Source: CAD feature listing. Evaluate the final solid. Frame: model axes, mm. Face numbers are marked on the shaded views. A direction names the side the tool comes from. Give positions to 0.01 mm unless a question says otherwise; leave off trailing zeros. Order: outer loops, then holes, each group sorted by start corner. A loop starts at its lowest first (then second) coordinate and runs counter-clockwise, first axis right, second up. Notation, with made-up numbers: (4, 61) - (35, 61) arc R26 ccw to (35, 81) - close; hole circle Ø4 at (56.25, -15.75). An arc over 180 degrees is marked (long way). Answer as CSV lines item,"result".
```python
from build123d import *
from build123d import SkipClean  # not in build123d's __all__

# Parameters (mm, degrees)
F3_DEPTH = 3.175
F4_DEPTH = 31.75
F5_DEPTH = 3.175
F6_DEPTH = 3.175


# Not quite as in the source:
# - a length typed as a fraction of an inch, garbled in the dataset ("3 / 203.2 mm" for 3/8 in), is restored


with BuildPart() as f3:
    # F2 (on Front) → F3 (new body)
    with BuildSketch(Plane.XZ):
        with BuildLine():
            Line((-3.175, 23.5998841364), (-3.175, 20.3918067186))
            ThreePointArc((-3.175, 20.3918067186), (-1.5922460699, 20.5759849996), (0, 20.6375))
            Line((0, 20.6375), (0, 23.8125))
            ThreePointArc((0, 23.8125), (-1.591055507, 23.7592865765), (-3.175, 23.5998841364))
        make_face()
        with BuildLine():
            ThreePointArc((20.6375, 0), (-13.4235305294, -15.6753065161), (-3.175, 20.3918067186))
            Line((-3.175, 20.3918067186), (-3.175, 23.5998841364))
            ThreePointArc((-3.175, 23.5998841364), (-15.6753065161, -17.9253987926), (23.8125, 0))
            ThreePointArc((23.8125, 0), (16.837980227, 16.837980227), (0, 23.8125))
            Line((0, 23.8125), (0, 20.6375))
            ThreePointArc((0, 20.6375), (14.5929161967, 14.5929161967), (20.6375, 0))
        make_face()
    extrude(amount=-F3_DEPTH)

    # F2 (on Front) → F4 (join)
    with BuildSketch(Plane.XZ):
        with BuildLine():
            ThreePointArc((0, 20.6375), (-1.5922460699, 20.5759849996), (-3.175, 20.3918067186))
            ThreePointArc((-3.175, 20.3918067186), (-13.4235305294, -15.6753065161), (20.6375, 0))
            ThreePointArc((20.6375, 0), (14.5929161967, 14.5929161967), (0, 20.6375))
        make_face()
    extrude(amount=F4_DEPTH)

    # F2 (on Front) → F5 (join)
    with BuildSketch(Plane.XZ):
        with BuildLine():
            Line((-3.175, 23.5998841364), (-3.175, 20.3918067186))
            ThreePointArc((-3.175, 20.3918067186), (-1.5922460699, 20.5759849996), (0, 20.6375))
            Line((0, 20.6375), (0, 23.8125))
            ThreePointArc((0, 23.8125), (-1.591055507, 23.7592865765), (-3.175, 23.5998841364))
        make_face()
    with SkipClean():  # cleaning this boolean's faces spoils the solid; the shape is the same uncleaned
        extrude(amount=F5_DEPTH)

    # F2 (on Front) → F6 (join)
    with BuildSketch(Plane.XZ):
        with BuildLine():
            ThreePointArc((0, 20.6375), (-1.5922460699, 20.5759849996), (-3.175, 20.3918067186))
            ThreePointArc((-3.175, 20.3918067186), (-13.4235305294, -15.6753065161), (20.6375, 0))
            ThreePointArc((20.6375, 0), (14.5929161967, 14.5929161967), (0, 20.6375))
        make_face()
        with BuildLine():
            Line((-3.175, 23.5998841364), (-3.175, 20.3918067186))
            ThreePointArc((-3.175, 20.3918067186), (-1.5922460699, 20.5759849996), (0, 20.6375))
            Line((0, 20.6375), (0, 23.8125))
            ThreePointArc((0, 23.8125), (-1.591055507, 23.7592865765), (-3.175, 23.5998841364))
        make_face()
    with SkipClean():  # cleaning this boolean's faces spoils the solid; the shape is the same uncleaned
        extrude(amount=-F6_DEPTH)


solid = f3.part
```
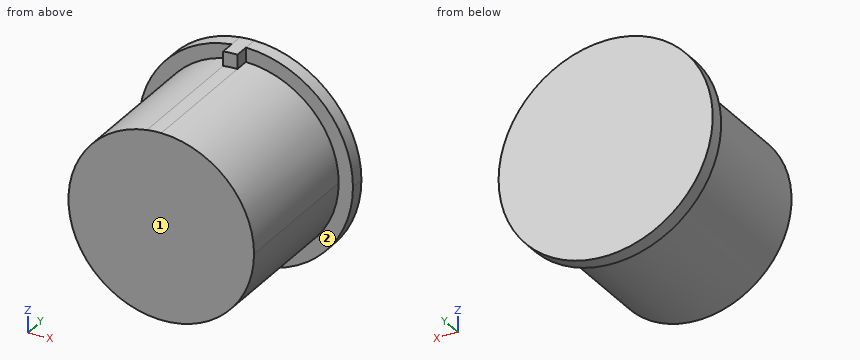
(1) Access query for the marked faces 1 and 2. Directions: +Z, -Z, +X, -X, +Y, -Y. A direction counts if a zero-diameter tool reaches every point of the face in a straight line with its end or side. Return the directions, or none.
Completed:
face 1,"+Z, -Z, +X, -X, -Y"
face 2,"-Y"
(2) Cut plane B-B (x = -19.5). Return loops of the section in (y, z) (3 decimals).
Completed:
outline,"(-31.75, -6.757) - (0, -6.757) - (0, -13.667) - (3.175, -13.667) - (3.175, 13.667) - (0, 13.667) - (0, 6.757) - (-31.75, 6.757) - close"
(3) Ray query, line 1 (Y direction, x = -18, z = -10.5) (3 decimals); line 2 (Z direction, x = -18.5, y = 1); line 3 (Z direction, x = 4, y = -20.5). Return the intervals inside material, ascending. Write a range as from..to.
Completed:
line 1,"0..3.175"
line 2,"-14.99..14.99"
line 3,"-20.25..20.25"
(4) Cut plane A-A (z = 17). Return loops of the section in (x, y) (3 decimals), then the cut area to 3 significant figures.
Completed:
outline,"(-16.674, 0) - (-11.701, 0) - (-11.701, -31.75) - (11.701, -31.75) - (11.701, 0) - (16.674, 0) - (16.674, 3.175) - (-16.674, 3.175) - close"
area,"849 mm²"
(5) Cut plane C-C (y = -17). Return loops of the section in (x, z) (1 decimal), then the cut area to 3 significant figures.
Completed:
outline,"circle Ø41.3 at (0, 0)"
area,"1,340 mm²"
(6) Contact query for flat-ended pins moving along their axis: pin 1 (1.6 mm diameter, centred on y = -2, z = 21.5, fed in from +X); pin 2 (4 mm diameter, centred on x = -17, y = -3.5, fed in from -Z); pin 3 (1.5 mm diameter, centred on y = -4.5, z = -3.5, fed in from -X). Output: stop coordinate, or through.
Completed:
pin 1,"x = 0"
pin 2,"z = -14.17"
pin 3,"x = -20.45"
